Geometry check sheet. Reference: the model listing, model coordinates, mm. Face numbers are marked on the shaded views. A direction names the side the tool comes from. Give positions to 0.01 mm unless a question says otherwise; leave off trailing zeros. Order: outer loops, then holes, each group sorted by start corner. A loop starts at its lowest first (then second) coordinate and runs counter-clockwise, first axis right, second up. Notation, with made-up numbers: M 7.5,61 L 45.5,61 A15 ccw 45.5,74 Z; hole C 52,-4 d9. An arc over 180 degrees is marked long. Answer as CSV lines item,"result". Start each with the question number.
Q1. Section check C-C, the plane y = -4.75. Record the boundary of the cut face in (x, z), then the cut area to 3 significant figures.
Q2. Mould release check, pull along Y, two halves, no side actions. Record for the marked faces 1, 2 and 3: +Y half, -Y half, draft (parallel to the pull), parting line (faces both ways), or undercut.
Q3. Section check A-A, the plane y = 0. Record the boundary of the cut face in (x, z), then the cut area to 3 significant figures.
Q4. Section check B-B, the plane y = -10. Record the boundary of the cut face in (x, z).
Q5. Thickness scan on line 1 (X direction, y = 0, z = 3.5); line 2 (X direction, y = 1.75, z = 1.25); line 3 (Y direction, x = 8.75, z = 1.25). Record the ranges inside material, lowest first.
Q6. Go/stop test with flat-tipped pins: pin 1 (2 mm diameter, centred on x = -6.5, z = 5, fed in from +Y); pin 2 (2 mm diameter, centred on y = -10, z = 6.5, fed in from -X); pin 3 (1 mm diameter, centred on x = 1, z = 4, fed in from -Y). Record where each tip stops, or that it passes through.
Q7. Section check D-D, the plane z = 7.25. Record the boundary of the cut face in (x, y).
Q8. Set-up check for the marked faces 4 and 5: record each of +Z, -Z, +X, -X, +Y, -Y from which the full face is reachable in a straight line by a thin tool's end or side.
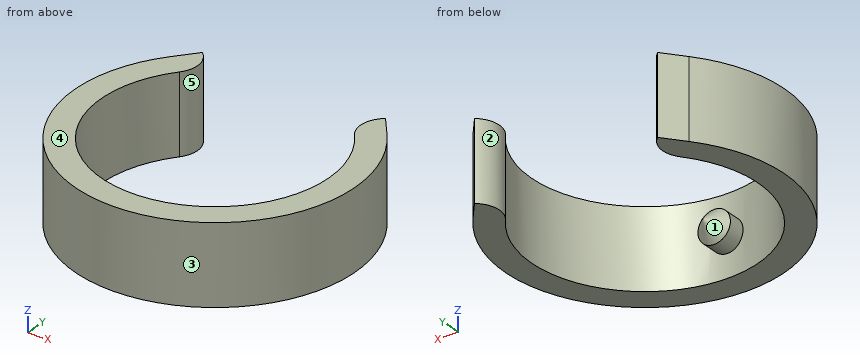
```python
from build123d import *

# Parameters (mm, degrees)
F1_DEPTH = 7.62
F3_R     = 1.5748
F4_DEPTH = 3.81
F5_SIZE  = 1.524


with BuildPart() as f1:
    # F0 (on Top) → F1 (new body)
    with BuildSketch(Plane.XY):
        with BuildLine():
            ThreePointArc((8.500466, 6.858), (0, -10.922), (-8.500466, 6.858))
            ThreePointArc((-8.500466, 6.858), (-7.951719, 8.722976), (-8.882435, 10.429736))
            Line((-8.882435, 10.429736), (-10.477318, 8.452884))
            ThreePointArc((-10.477318, 8.452884), (0, -13.462), (10.477318, 8.452884))
            Line((10.477318, 8.452884), (8.882435, 10.429736))
            ThreePointArc((8.882435, 10.429736), (7.951719, 8.722976), (8.500466, 6.858))
        make_face()
    extrude(amount=F1_DEPTH)

    # F3 (on offset) → F4 (join)
    with BuildSketch(Plane.XZ.offset(11.43)):
        with Locations((0, 3.81)):
            Circle(F3_R)
    extrude(amount=-F4_DEPTH)

    # F5
    f5_edges = [f1.edges().sort_by_distance(p)[0] for p in [
        (-1.5748, -7.62, 3.81),
    ]]
    chamfer(f5_edges, length=F5_SIZE)


solid = f1.part
```
Answer block:
1,outline,"M -12.6,0 L -9.84,0 L -9.84,7.62 L -12.6,7.62 Z; M 9.84,0 L 12.6,0 L 12.6,7.62 L 9.84,7.62 Z"
1,area,"42.1 mm2"
2,face 1,"+Y half"
2,face 2,"undercut"
2,face 3,"parting line"
3,outline,"M -13.46,0 L -10.92,0 L -10.92,7.62 L -13.46,7.62 Z; M 10.92,0 L 13.46,0 L 13.46,7.62 L 10.92,7.62 Z"
3,area,"38.7 mm2"
4,outline,"M -9.01,0 L -4.39,0 L -4.39,7.62 L -9.01,7.62 Z; C 0,3.81 d3.15; M 4.39,0 L 9.01,0 L 9.01,7.62 L 4.39,7.62 Z"
5,line 1,"x = -13.46 to -10.92, 10.92 to 13.46"
5,line 2,"x = -13.35 to -10.78, 10.78 to 13.35"
5,line 3,"y = -10.23 to -6.54, 6.54 to 10.32"
6,pin 1,"stops at y = -7.94"
6,pin 2,"stops at x = -10.01"
6,pin 3,"stops at y = -13.45"
7,outline,"M -10.48,8.45 A13.46 ccw long 10.48,8.45 L 8.88,10.43 A2.54 ccw 8.5,6.86 A10.92 cw long -8.5,6.86 A2.54 ccw -8.88,10.43 Z"
8,face 4,"+Z, +X, -X, +Y, -Y"
8,face 5,"+Z, -Z"
